Could you check a few things on this model? Use its own coordinates, in mm. Face numbers are marked on the shaded views. Give positions to 0.01 mm unless a question says otherwise; leave off trailing zeros. Loops run counter-clockwise (first coordinate to the right, second up) from the corner with the lowest first, then second, coordinate; pieces in that order, holes last. Notation, with made-up numbers: M 42.5,86.5 L 55.5,86.5 A29 cw 55.5,124.5 Z; hole C 74.5,50 d7. An arc over 180 degrees is marked long. Answer in a Markdown table with one row per item. Add a question column.
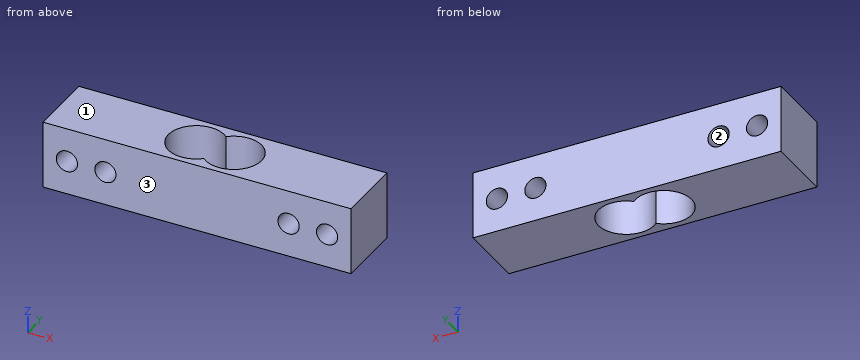
```python
from build123d import *

# Parameters (mm, degrees)
SKETCH1_W               = 58
SKETCH1_H               = 12.7
SKETCH1_R               = 2
BOSS_EXTRUDE1_DEPTH     = 12.75
CUT_EXTRUDE2_DEPTH      = 35.129935541
CUT_EXTRUDE2_DEPTH_BACK = 35.129935541


with BuildPart() as part:
    # Sketch1 → Boss-Extrude1 (new body)
    with BuildSketch(Plane(origin=(0, 0, 0), x_dir=(1, 0, 0), z_dir=(0, 1, 0))):
        Rectangle(SKETCH1_W, SKETCH1_H)
        with Locations(Location((-24.5, 0, 0), (0, 0, 270))):
            Circle(SKETCH1_R, mode=Mode.SUBTRACT)
        with Locations(Location((-17.25, 0, 0), (0, 0, 270))):
            Circle(SKETCH1_R, mode=Mode.SUBTRACT)
        with Locations(Location((24.5, 0, 0), (0, 0, 270))):
            Circle(SKETCH1_R, mode=Mode.SUBTRACT)
        with Locations(Location((17.25, 0, 0), (0, 0, 270))):
            Circle(SKETCH1_R, mode=Mode.SUBTRACT)
    extrude(amount=BOSS_EXTRUDE1_DEPTH)

    # Sketch2 → Cut-Extrude2 (cut, two sides: drawn at the far end of the back side and taken through both)
    with BuildSketch(Plane.XY.offset(6.35).offset(-CUT_EXTRUDE2_DEPTH_BACK)):
        with BuildLine():
            ThreePointArc((0, 10.265613705), (-8.775, 6.375), (0, 2.484386295))
            ThreePointArc((0, 2.484386295), (8.775, 6.375), (0, 10.265613705))
        make_face()
    extrude(amount=CUT_EXTRUDE2_DEPTH + CUT_EXTRUDE2_DEPTH_BACK, mode=Mode.SUBTRACT)


solid = part.part
```
Item 1: Suppose I cut it at B-B (z = 0). List the corners of the cut face in (x, y) for me (3 decimals).
Item 2: For P1, Ø2, axis at x = -5.5, y = 5, coming from the -Z side; P2, Ø4.5, axis at x = 17.25, z = 0, coming from the +Y side, each with a flat end and sliding along its axis, tell me the tip position at first contact or that it passes through.
Item 3: Suppose I cut it at C-C (y = 4). List the corners of the cut face in (x, z) for me, then the cut area to 3 significant figures.
Item 4: If we mould it in two halves opening along Z, with no side actions, what happens to the marked faces 1, 2 and 3? For each: +Z half, -Z half, draft (parallel to the pull), parting line (faces both ways), or undercut.
Item 5: Suppose I cut it at A-A (x = 24.5). List the corners of the cut face in (y, z) for me.
Item 6: I need wall thicknesses on L1, parallel to X at y = 7.25, z = 0; L2, parallel to X at y = 6, z = -0.5; L3, parallel to Y at x = -3.5, z = -5. Which ranges of each line are inside material? Lowest first, please.
Item 7: Suppose I cut it at D-D (x = 7). List the corners of the cut face in (y, z) for me.
Values found:
| question | item | result |
|---|---|---|
| 1 | outline | M -29,0 L -26.5,0 L -26.5,12.75 L -29,12.75 Z; M -22.5,0 L -19.25,0 L -19.25,12.75 L -22.5,12.75 Z; M -15.25,0 L 15.25,0 L 15.25,12.75 L -15.25,12.75 Z; M 19.25,0 L 22.5,0 L 22.5,12.75 L 19.25,12.75 Z; M 26.5,0 L 29,0 L 29,12.75 L 26.5,12.75 Z; hole M 0,2.484 A5.25 ccw long 0,10.266 A5.25 ccw long Z |
| 2 | P1 | through |
| 2 | P2 | y = 12.75 |
| 3 | outline | M -29,-6.35 L -8.21,-6.35 L -8.21,6.35 L -29,6.35 Z; M 8.21,-6.35 L 29,-6.35 L 29,6.35 L 8.21,6.35 Z; hole C -24.5,0 d4; hole C -17.25,0 d4; hole C 17.25,0 d4; hole C 24.5,0 d4 |
| 3 | area | 478 mm² |
| 4 | face 1 | +Z half |
| 4 | face 2 | undercut |
| 4 | face 3 | draft |
| 5 | outline | M 0,-6.35 L 12.75,-6.35 L 12.75,-2 L 0,-2 Z; M 0,2 L 12.75,2 L 12.75,6.35 L 0,6.35 Z |
| 6 | L1 | -29 to -26.5, -22.5 to -19.25, -15.25 to -8.7, 8.7 to 15.25, 19.25 to 22.5, 26.5 to 29 |
| 6 | L2 | -29 to -26.44, -22.56 to -19.19, -15.31 to -8.76, 8.76 to 15.31, 19.19 to 22.56, 26.44 to 29 |
| 6 | L3 | 0 to 1.13, 11.62 to 12.75 |
| 7 | outline | M 0,-6.35 L 2.44,-6.35 L 2.44,6.35 L 0,6.35 Z; M 10.31,-6.35 L 12.75,-6.35 L 12.75,6.35 L 10.31,6.35 Z |
